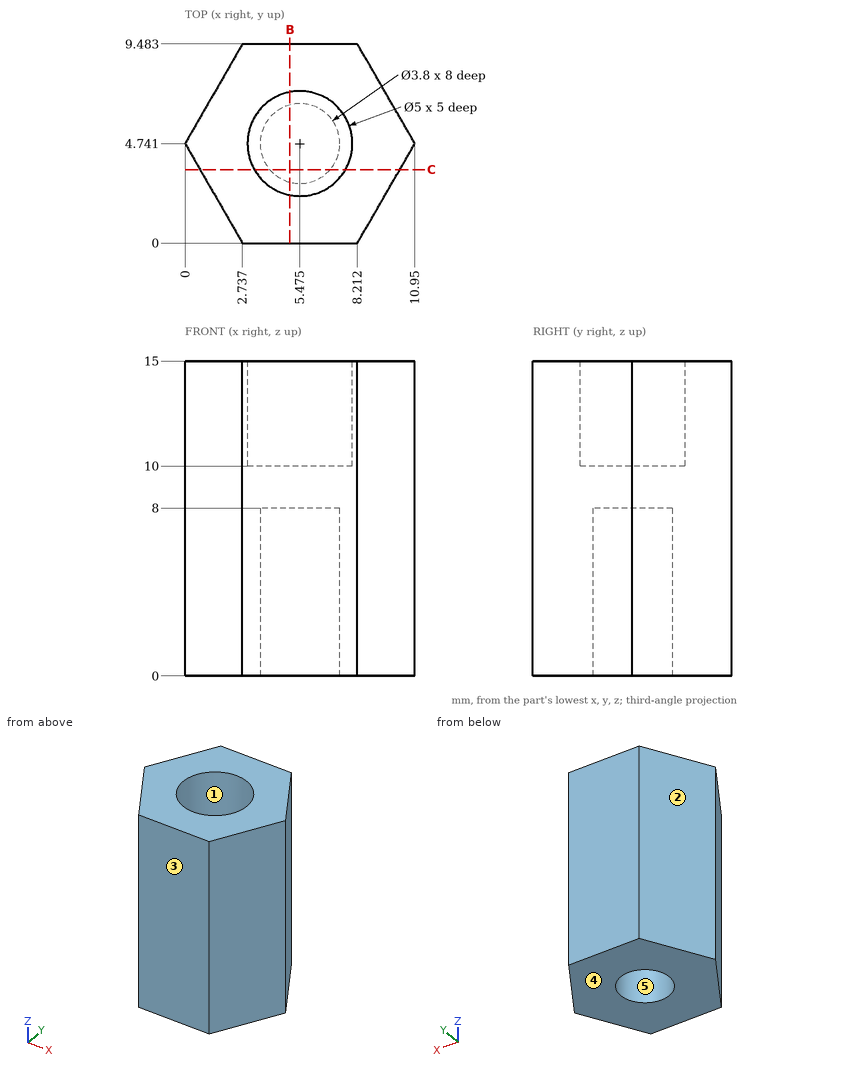
Drawing for the job (mm, zero at the part's lowest x, y, z). A direction names the side the tool comes from. Give positions to 0.01 mm unless a question says otherwise; leave off trailing zeros. Order: outer loops, then holes, each group sorted by start corner. A loop starts at its lowest first (then second) coordinate and runs counter-clockwise, first axis right, second up. Notation, with made-up numbers: (-35, -31) - (-26, -31) arc R28 ccw to (-26, -9) - close; hole circle Ø6 at (29.25, 37). An arc over 180 degrees is marked (long way). Write item = value, one per line. Start each with the question number.
1. Which spindle directions (+Z, -Z, +X, -X, +Y, -Y) get a long thin tool onto all of the face, cutting with end or side? Do the marked faces 4 and 5. Say none if no direction does.
2. Cut at B-B, the plane x = 5. List the corners of the cut face in (y, z) (1 decimal).
3. Cut at C-C, the plane y = 3.5. List the corners of the cut face in (x, z) (1 decimal).
4. Two-plate mould, pull along Y, no slides. Class the marked faces 1, 2 and 3: pulls with the +Y half, pulls with the -Y half, needs draft (parallel to the pull), parting line crosses it, or undercut.
5. Probe line 1 along Y through (x, z) = (5.5, 10.75); line 2 along Z through (x, y) = (6.5, 5.5); line 3 along Y through (x, z) = (5.75, 5). List the from-to ranges inside material, lowest first.
Taken from the geometry:
q1.face_4 = -Z, +X, -X, +Y, -Y
q1.face_5 = -Z
q2.outline = (0, 0) - (2.9, 0) - (2.9, 8) - (6.6, 8) - (6.6, 0) - (9.5, 0) - (9.5, 15) - (7.2, 15) - (7.2, 10) - (2.3, 10) - (2.3, 15) - (0, 15) - close
q3.outline = (0.7, 0) - (4, 0) - (4, 8) - (6.9, 8) - (6.9, 0) - (10.2, 0) - (10.2, 15) - (7.6, 15) - (7.6, 10) - (3.3, 10) - (3.3, 15) - (0.7, 15) - close
q4.face_1 = undercut
q4.face_2 = pulls with the +Y half
q4.face_3 = pulls with the -Y half
q5.line_1 = 0 to 2.24, 7.24 to 9.48
q5.line_2 = 8 to 10
q5.line_3 = 0 to 2.86, 6.62 to 9.48
